Geometry: final body of the model. Coordinates: model frame, mm. A direction names the side the tool comes from. Round coordinates to 2 decimals unless told otherwise and drop trailing zeros. Order: outer loops, then holes, each group sorted by start corner. A loop starts at its lowest first (then second) coordinate and runs counter-clockwise, first axis right, second up. Notation, with made-up numbers: (-26.75, 80.25) -> (24.25, 80.25) arc R28 ccw to (24.25, 108.25) -> close; hole circle Ø5 at (85, 68). An arc over 180 degrees is marked (long way). Put each result on its own line as item: value.
Autodesk Inventor part; units mm, degrees
ref_plane "YZ Plane" through (0, 0, 0) normal (1, 0, 0) x (0, 1, 0)
ref_plane "XZ Plane" through (0, 0, 0) normal (0, 1, 0) x (-1, 0, 0)
ref_plane "XY Plane" through (0, 0, 0) normal (0, 0, 1) x (1, 0, 0)
sketch "Sketch1" plane through (0, 0, 0) normal (0, 0, 1) x (1, 0, 0)
  circle A0 centre (0, 0) radius 4.5
  dimension "d0" = 9
extrude "Extrusion1" add sketch "Sketch1" along normal blind 6.8
sketch "Sketch2" plane through (0, 0, 6.8) normal (0, 0, 1) x (1, 0, 0)
  line L0 (-1.7898, 3.1) -> (1.7898, 3.1)
  line L1 (1.7898, 3.1) -> (3.5796, 0)
  line L2 (3.5796, 0) -> (1.7898, -3.1)
  line L3 (1.7898, -3.1) -> (-1.7898, -3.1)
  line L4 (-1.7898, -3.1) -> (-3.5796, 0)
  line L5 (-3.5796, 0) -> (-1.7898, 3.1)
  point P0 (0, 0)
  point P1 (0, 3.1)
  point P2 (0, -3.1)
  dimension "d3" = 6.2
  dimension "d4" = 6.2
extrude "Extrusion2" cut sketch "Sketch2" against normal blind 5.3
sketch "Sketch3" plane through (0, 0, 0) normal (0, 0, -1) x (-1, 0, 0)
  circle A0 centre (0, 0) radius 1.25
  dimension "d7" = 2.5
sketch "Sketch4" plane through (0, 0, 1.5) normal (0, 0, 1) x (1, 0, 0)
  circle A0 centre (0, 0) radius 3.1
  dimension "d8" = 6.2
loft "Loft1" cut profiles "Sketch4", "Sketch3"
sketch "Sketch5" plane through (0, 0, 0) normal (0, 1, 0) x (-1, 0, 0)
  line L0 (-4.5, 0) -> (4.5, 0)
  line L1 (2.5, 0) -> (4.5, 2.5)
  line L2 (4.5, 2.5) -> (4.5, 0)
  line L3 (4.5, 0) -> (2.5, 0)
  line L4 (0, -0.5) -> (0, 3)
  point P0 (0, 0)
  dimension "d14" = 2.5
  dimension "d15" = 2
revolve "Revolution1" cut sketch "Sketch5" angle 360 about axis through (0, 0, -10) along (0, 0, 1)
equation "\"d4\" = d3"
properties part number "mouthcover"
1. Material intervals for probe 1 along Y at (x, z) = (0, 1.75); probe 2 along X at (y, z) = (0.5, 2); probe 3 along X at (y, z) = (-0.75, 0.5), sorted ascending.
Ans:
probe 1: -3.9 to -3.1, 3.1 to 3.9
probe 2: -4.07 to -3.29, 3.29 to 4.07
probe 3: -2.8 to -1.71, 1.71 to 2.8
2. Set-up query: faces 5 (the face through (-3.26, 0.24, 1.5)), 6 (the face through (1.1, -1.1, 0)). Return all of +Z, -Z, +X, -X, +Y, -Y with unobstructed straight access to the full face (end or side cutting, diameter ignored); none if empty.
Ans:
face 5: +Z
face 6: -Z, +X, -X, +Y, -Y
3. Contact query for flat-ended pins moving along their axis: P1, Ø1.5, axis at x = 1.5, z = 3.5, coming from the +Y side; P2, Ø4, axis at x = -2, y = 1.5, coming from the +Z side; P3, Ø1.1, axis at x = -1, z = 5, coming from the -Y side; P4, Ø1, axis at x = 1.5, y = -2.5, coming from the +Z side. Output: stop coordinate, or through.
Ans:
P1: y = 4.44
P2: z = 6.8
P3: y = -4.48
P4: z = 1.5
4. Cut plane A-A on z = 2.75. Return loops of the section in (x, y), and give its area (3 significant figures).
Ans:
outline: circle Ø9 at (0, 0); hole (-3.58, 0) -> (-1.79, -3.1) -> (1.79, -3.1) -> (3.58, 0) -> (1.79, 3.1) -> (-1.79, 3.1) -> close
area: 30.3 mm²
5. Draft query along X for faces 1 (the face through (0, 3.1, 4)), 2 (the face through (2.697, -1.528, 4.187)), 3 (the face through (3, -2, 6.8)), 4 (the face through (-2.504, -0.789, 0.156)). Return one class per face: +X half, -X half, draft (parallel to the pull), parting line (faces both ways), or undercut.
Ans:
face 1: undercut
face 2: undercut
face 3: draft
face 4: parting line
